The model under review builds one solid part; all positions refer to its coordinate system, in mm. A direction names the side the tool comes from. Give positions to 0.01 mm unless a question says otherwise; leave off trailing zeros. Loops run counter-clockwise (first coordinate to the right, second up) from the corner with the lowest first, then second, coordinate; pieces in that order, holes last. Notation, with made-up numbers: M -4.75,-8.75 L 23.25,-8.75 A16 ccw 23.25,19.25 Z; hole C 77,39.25 d2. An arc over 180 degrees is marked long. Return JSON: item names as keys, results as strings. Group by question number.
```python
from build123d import *

# Parameters (mm, degrees)
SKETCH2_R           = 17.5
BOSS_EXTRUDE1_DEPTH = 49
CUT_EXTRUDE1_START  = -49
SKETCH3_R           = 7
CUT_EXTRUDE1_DEPTH  = 49


# Read off the part's stored shape, not the designer's step: M6 Tapped Hole1
with BuildPart() as part:
    # Sketch2 → Boss-Extrude1 (new, symmetric)
    with BuildSketch(Plane(origin=(0, 0, 0), x_dir=(0, 0, -1), z_dir=(1, 0, 0))):
        Circle(SKETCH2_R)
    extrude(amount=BOSS_EXTRUDE1_DEPTH, both=True)

    # Sketch3 → Cut-Extrude1 (cut)
    with BuildSketch(Plane(origin=(49, 0, 0), x_dir=(0, 0, -1), z_dir=(1, 0, 0)).offset(CUT_EXTRUDE1_START)):
        Circle(SKETCH3_R)
    extrude(amount=CUT_EXTRUDE1_DEPTH, mode=Mode.SUBTRACT)

    # M6 Tapped Hole1 outline → M6 Tapped Hole1 (revolve, cut)
    with BuildSketch(Plane(origin=(0, -7.5, -10), x_dir=(0, 1, 0), z_dir=(0, 0, -1))):
        Polygon((0, 49), (0, 31), (2.5, 32.502151548), (2.5, 48.475), (3.025, 49), align=None)
    m6_tapped_hole1 = revolve(axis=Axis((0, -7.5, -10), (1, 0, 0)), mode=Mode.SUBTRACT)

    # M6 Tapped Hole1 2 outline → M6 Tapped Hole1 2 (revolve, cut)
    with BuildSketch(Plane(origin=(0, 7.5, 10), x_dir=(0, 1, 0), z_dir=(0, 0, -1))):
        Polygon((0, 49), (0, 31), (2.5, 32.502151548), (2.5, 48.475), (3.025, 49), align=None)
    m6_tapped_hole1_2 = revolve(axis=Axis((0, 7.5, 10), (1, 0, 0)), mode=Mode.SUBTRACT)

    # M6 Tapped Hole1 3 outline → M6 Tapped Hole1 3 (revolve, cut)
    with BuildSketch(Plane(origin=(0, -7.5, 10), x_dir=(0, 1, 0), z_dir=(0, 0, -1))):
        Polygon((0, 49), (0, 31), (2.5, 32.502151548), (2.5, 48.475), (3.025, 49), align=None)
    m6_tapped_hole1_3 = revolve(axis=Axis((0, -7.5, 10), (1, 0, 0)), mode=Mode.SUBTRACT)

    # M6 Tapped Hole1 4 outline → M6 Tapped Hole1 4 (revolve, cut)
    with BuildSketch(Plane(origin=(0, 7.5, -10), x_dir=(0, 1, 0), z_dir=(0, 0, -1))):
        Polygon((0, 49), (0, 31), (2.5, 32.502151548), (2.5, 48.475), (3.025, 49), align=None)
    m6_tapped_hole1_4 = revolve(axis=Axis((0, 7.5, -10), (1, 0, 0)), mode=Mode.SUBTRACT)

    # Mirror1: M6 Tapped Hole1, M6 Tapped Hole1 2, M6 Tapped Hole1 3, M6 Tapped Hole1 4 across plane
    add(m6_tapped_hole1.mirror(Plane(origin=(0, 0, 0), x_dir=(0, 0, 1), z_dir=(1, 0, 0))), mode=Mode.SUBTRACT)
    add(m6_tapped_hole1_2.mirror(Plane(origin=(0, 0, 0), x_dir=(0, 0, 1), z_dir=(1, 0, 0))), mode=Mode.SUBTRACT)
    add(m6_tapped_hole1_3.mirror(Plane(origin=(0, 0, 0), x_dir=(0, 0, 1), z_dir=(1, 0, 0))), mode=Mode.SUBTRACT)
    add(m6_tapped_hole1_4.mirror(Plane(origin=(0, 0, 0), x_dir=(0, 0, 1), z_dir=(1, 0, 0))), mode=Mode.SUBTRACT)


solid = part.part
```
(1) Add section C-C (x = -33.5). Write out the cut boundary in (y, z).
(2) Add section D-D (x = 17). Write out the cut boundary in (y, z), and give its area (3 significant figures).
(3) For pin 1 (12 mm diameter, centred on x = 26.5, z = -11.5, fed in from +Y); pin 2 (3 mm diameter, centred on x = 36.5, y = -7.5, fed in from -Z); pin 3 (3 mm diameter, centred on y = -7.5, z = 10, fed in from +X); pin 4 (5 mm diameter, centred on y = 6.5, z = -8, fed in from -X), all flat-tipped, find the tip position at first contact; note any pin that passes through.
(4) For faces 3 (the cylindrical face through (-41, 9, -12)), 4 (the cylindrical face through (41, 9, -12)), list the 3-axis set-ups (+Z, -Z, +X, -X, +Y, -Y) from which the entire face can be reached by the end or side of a thin tool; tool diameter is ignored.
(5) For probe 1 along Z at (x, y) = (-35, 8.5); probe 2 along Y at (x, z) = (18, 0); probe 3 along Y at (x, z) = (35, 8), list the stretches that pass through material, from the lowest coordinate up.
(6) Add section A-A (y = 0). Write out the cut boundary in (x, z), and give its area (3 significant figures).
(7) Mouldability with a two-part tool opening along Y and no side actions: class faces 1 (the cylindrical face through (0.686, -10.648, 13.887)), 2 (the conical face through (31.26, -7.56, 10.43)) as released by +Y, released by -Y, zero draft, split by the parting line, or undercut.
Verdict:
{
 "1": {"outline": "C 0,0 d35; hole C -7.5,-10 d5; hole C -7.5,10 d5; hole C 7.5,-10 d5; hole C 7.5,10 d5"},
 "2": {"outline": "C 0,0 d35; hole C 0,0 d14", "area": "808 mm²"},
 "3": {"pin 1": "stops at y = 16.61", "pin 2": "stops at z = -16.44", "pin 3": "stops at x = 31.9", "pin 4": "stops at x = -49"},
 "4": {"face 3": "-X", "face 4": "+X"},
 "5": {"probe 1": "z = -15.3 to -12.29, -7.71 to 7.71, 12.29 to 15.3", "probe 2": "y = -17.5 to -7, 7 to 17.5", "probe 3": "y = -15.56 to -9, -6 to 6, 9 to 15.56"},
 "6": {"outline": "M -49,-17.5 L 49,-17.5 L 49,-7 L 0,-7 L 0,7 L 49,7 L 49,17.5 L -49,17.5 Z", "area": "2,740 mm²"},
 "7": {"face 1": "split by the parting line", "face 2": "undercut"}
}
